Geometry check sheet. Reference: the model listing, model coordinates, mm. A direction names the side the tool comes from. Coordinates: 2 decimals unless noted, no trailing zeros. Loops run counter-clockwise (first coordinate to the right, second up) from the corner with the lowest first, then second, coordinate; pieces in that order, holes last. Notation, with made-up numbers: M 47,-35 L 64,-35 A17 ccw 64,-23 Z; hole C -7.5,57.5 d7. An arc over 180 degrees is marked long. One line per question, with ' | ' between items. Start each with the question number.
from build123d import *

# Parameters (mm, degrees)
BOSS_EXTRUDE1_DEPTH = 40
SKETCH2_R           = 15.049999999999999
CUT_EXTRUDE1_DEPTH  = 40
FILLET3_R           = 18.700000000000003
FILLET4_R           = 18.7
FILLET5_R           = 18.7
FILLET6_R           = 18.7
SKETCH4_R           = 15.049999999999999
CUT_EXTRUDE2_DEPTH  = 30


with BuildPart() as part:
    # Sketch1 → Boss-Extrude1 (new body)
    with BuildSketch(Plane.XY):
        with BuildLine():
            Line((-21.97749224689504, -20.420328952729147), (-56.618508398272695, -40.420328952728944))
            Line((-56.618508398272695, -40.420328952728944), (-74.08417498363409, -10.168907038824594))
            Line((-74.08417498363409, -10.168907038824594), (-22.896447841875652, 19.38434100567434))
            ThreePointArc((-22.896447841875652, 19.38434100567434), (1.84e-15, 30), (22.89644784187566, 19.384341005674337))
            Line((22.89644784187566, 19.384341005674337), (74.08417498363407, -10.168907038825086))
            Line((74.08417498363407, -10.168907038825086), (56.61850839827255, -40.42032895272918))
            Line((56.61850839827255, -40.42032895272918), (21.97749224689504, -20.42032895272915))
            ThreePointArc((21.97749224689504, -20.42032895272915), (-4.82e-15, -29.999999999999996), (-21.97749224689504, -20.420328952729147))
        make_face()
    extrude(amount=BOSS_EXTRUDE1_DEPTH)

    # Sketch2 → Cut-Extrude1 (cut)
    with BuildSketch(Plane(origin=(59.96639714989796, -34.62161553682567, 0), x_dir=(0, 0, -1), z_dir=(0.8660254037844382, -0.5000000000000009, 0))):
        with Locations(Location((-20, 10.769889082110701, 0), (0, 0, 90))):
            Circle(SKETCH2_R)
    cut_extrude1 = extrude(amount=-CUT_EXTRUDE1_DEPTH, mode=Mode.SUBTRACT)

    # Mirror1: Cut-Extrude1 across plane
    add(cut_extrude1.mirror(Plane(origin=(0, 0, 0), x_dir=(0, 0, 1), z_dir=(1, 0, 0))), mode=Mode.SUBTRACT)

    # Fillet3
    fillet3_edges = [part.edges().sort_by_distance(p)[0] for p in [
        (39.298000322583796, -30.420328952729164, 40),
    ]]
    fillet(fillet3_edges, radius=FILLET3_R)

    # Fillet4
    # the kernel refuses this fillet: 18.7 mm, written as the material it takes off along each edge
    with BuildSketch(Plane(origin=(-17.590239785046823, 42.759341005674386, 40), x_dir=(0, 0, -1), z_dir=(0.866025403784438, -0.5000000000000011, 0))) as fillet4_piece_1_section:
        with BuildLine():
            CenterArc((FILLET4_R, -FILLET4_R), FILLET4_R, 90, 89.99999999999997)
            Line((0, -FILLET4_R), (0, 0))
            Line((0, 0), (FILLET4_R, 0))
        make_face()
    fillet4_piece_1 = extrude(amount=152.6064960889987, mode=Mode.PRIVATE)
    fillet4_piece_1 = fillet4_piece_1 - Plane(origin=(2.66e-15, 5.33e-15, 35.12262503865641), x_dir=(-0.7632149280625219, 0.6461447001891446, 0), z_dir=(0, 0, -1)) * Cylinder(29.999999999999996, 381, mode=Mode.PRIVATE)
    add(fillet4_piece_1, mode=Mode.SUBTRACT)
    with BuildSketch(Plane(origin=(18.509195380027606, 2.9546710472706206, 0), x_dir=(-0.49999999999999495, 0.8660254037844416, 0), z_dir=(-0.8660254037844416, -0.499999999999995, 0))) as fillet4_piece_2_section:
        with BuildLine():
            CenterArc((FILLET4_R, -FILLET4_R), FILLET4_R, 90, 90)
            Line((-2.49e-15, -FILLET4_R), (0, 0))
            Line((0, 0), (FILLET4_R, 0))
        make_face()
    fillet4_piece_2 = extrude(amount=133.50000000000003, mode=Mode.PRIVATE)
    fillet4_piece_2 = fillet4_piece_2 - Plane(origin=(8.9e-16, 5.33e-15, 4.238028125601217), x_dir=(0.7325830748965012, -0.6806776317576385, 0), z_dir=(0, 0, -1)) * Cylinder(30, 342, mode=Mode.PRIVATE)
    add(fillet4_piece_2, mode=Mode.SUBTRACT)
    with BuildSketch(Plane(origin=(97.10519602519503, -63.795328952729214, 0), x_dir=(0.5000000000000009, 0.8660254037844382, 0), z_dir=(-0.8660254037844382, 0.5000000000000009, 0))) as fillet4_piece_3_section:
        with BuildLine():
            CenterArc((FILLET4_R, -FILLET4_R), FILLET4_R, 90, 90)
            Line((0, -FILLET4_R), (0, 0))
            Line((0, 0), (FILLET4_R, 0))
        make_face()
    fillet4_piece_3 = extrude(amount=133.49999999999997, mode=Mode.PRIVATE)
    fillet4_piece_3 = fillet4_piece_3 - Plane(origin=(8.9e-16, 5.33e-15, 4.238027498797153), x_dir=(0.7325830748965012, -0.6806776317576385, 0), z_dir=(0, 0, -1)) * Cylinder(30, 342, mode=Mode.PRIVATE)
    add(fillet4_piece_3, mode=Mode.SUBTRACT)

    # Fillet5
    # the kernel refuses this fillet: 18.7 mm, written as the material it takes off along each edge
    with BuildSketch(Plane(origin=(-114.57086261055673, -33.54390703882436, 0), x_dir=(0.4999999999999949, -0.8660254037844416, 0), z_dir=(0.8660254037844416, 0.49999999999999484, 0))) as fillet5_piece_1_section:
        with BuildLine():
            CenterArc((FILLET5_R, -FILLET5_R), FILLET5_R, 90, 90)
            Line((0, -FILLET5_R), (0, 0))
            Line((0, 0), (FILLET5_R, 0))
        make_face()
    fillet5_piece_1 = extrude(amount=152.6064960889985, mode=Mode.PRIVATE)
    fillet5_piece_1 = fillet5_piece_1 - Plane(origin=(8.9e-16, 5.33e-15, 4.361975698368192), x_dir=(0.7325830748965012, -0.6806776317576385, 0), z_dir=(0, 0, -1)) * Cylinder(30, 381, mode=Mode.PRIVATE)
    with BuildSketch(Plane(origin=(18.509195380027606, 2.954671047270619, 40), x_dir=(1e-17, -2e-17, -1), z_dir=(-0.8660254037844416, -0.499999999999995, 0))) as fillet5_piece_2_section:
        with BuildLine():
            CenterArc((FILLET5_R, -FILLET5_R), FILLET5_R, 90, 90)
            Line((-4.8e-16, -FILLET5_R), (0, 0))
            Line((0, 0), (FILLET5_R, 0))
        make_face()
    fillet5_piece_2 = extrude(amount=133.50000000000003, mode=Mode.PRIVATE)
    fillet5_piece_2 = fillet5_piece_2 - Plane(origin=(8.9e-16, 5.33e-15, 35.76197179193409), x_dir=(0.7325830748965012, -0.6806776317576385, 0), z_dir=(0, 0, -1)) * Cylinder(30, 342, mode=Mode.PRIVATE)
    with BuildSketch(Plane(origin=(-17.590239785046823, 42.759341005674386, 0), x_dir=(0, 0, 1), z_dir=(0.866025403784438, -0.5000000000000011, 0))) as fillet5_piece_3_section:
        with BuildLine():
            CenterArc((FILLET5_R, FILLET5_R), FILLET5_R, 180.00000000000003, 90)
            Line((-3.55e-15, FILLET5_R), (0, 0))
            Line((0, 0), (FILLET5_R, 0))
        make_face()
    fillet5_piece_3 = extrude(amount=152.6064960889987, mode=Mode.PRIVATE)
    fillet5_piece_3 = fillet5_piece_3 - Plane(origin=(8.9e-16, 5.33e-15, 4.877369917658315), x_dir=(0.7325830748965012, -0.6806776317576385, 0), z_dir=(0, 0, -1)) * Cylinder(30, 381, mode=Mode.PRIVATE)
    add([fillet5_piece_1, fillet5_piece_2, fillet5_piece_3], mode=Mode.SUBTRACT)

    # Fillet6
    # the kernel refuses this fillet: 18.7 mm, written as the material it takes off along each edge
    with BuildSketch(Plane(origin=(-114.57086261055673, -33.54390703882436, 40), x_dir=(0.4999999999999949, -0.8660254037844416, 0), z_dir=(0.8660254037844416, 0.49999999999999484, 0))) as fillet6_piece_1_section:
        with BuildLine():
            CenterArc((FILLET6_R, FILLET6_R), FILLET6_R, 180, 90)
            Line((0, FILLET6_R), (0, 0))
            Line((0, 0), (FILLET6_R, 0))
        make_face()
    fillet6_piece_1 = extrude(amount=152.6064960889985, mode=Mode.PRIVATE)
    fillet6_piece_1 = fillet6_piece_1 - Plane(origin=(8.9e-16, 5.33e-15, 35.63802430163197), x_dir=(0.7325830748965012, -0.6806776317576385, 0), z_dir=(0, 0, -1)) * Cylinder(30, 381, mode=Mode.PRIVATE)
    add(fillet6_piece_1, mode=Mode.SUBTRACT)

    # Sketch4 → Cut-Extrude2 (cut)
    with BuildSketch(Plane(origin=(0, 0, 0), x_dir=(-1, 0, 0), z_dir=(0, 0, -1))):
        Circle(SKETCH4_R)
    extrude(amount=-CUT_EXTRUDE2_DEPTH, mode=Mode.SUBTRACT)


solid = part.part
1. Draft check along X on faces 1 (the cylindrical face through (-52.079, -3.138, 33.935)), 2 (the flat face through (0, 0, 30)), 3 (the flat face through (48.132, 4.815, 19.982)). Enter one of: +X half, -X half, draft (parallel to the pull), parting line (faces both ways), or undercut.
2. Thickness scan on line 1 (X direction, y = -16, z = 4.5); line 2 (X direction, y = 2, z = 20.5); line 3 (Y direction, x = 0, z = 12). Record the ranges inside material, lowest first.
3. Depth check by flat-ended pin: pin 1 Ø6 at (x, z) = (-28.5, 30) entering from -Y; pin 2 Ø12 at (x, z) = (1, 24.5) entering from -Y; pin 3 Ø15 at (x, y) = (-3.5, 0.5) entering from -Z; pin 4 Ø10 at (x, y) = (-27, 15.5) entering from -Z. Enter the tip coordinate at first touch or a pass-through.
4. Sectioned sample at D-D (y = 0). State how many separate pieces and enclosed holes the cut face has, and give its area (3 significant figures).
5. Sectioned sample at C-C (z = 33). Record the cut outline in (x, y).
6. Sectioned sample at A-A (z = 13.5). Record the cut outline in (x, y), and give its area (3 significant figures).
7. Tool access check on faces 4 (the cylindrical face through (-40.967, -25.71, 33.935)), 5 (the cylindrical face through (3.263, -14.692, 14.79)), 6 (the cylindrical face through (41.6, -25.77, 5.78)), 7 (the flat face through (39.54, -30.56, 19.98)). Record the directions out of +Z, -Z, +X, -X, +Y, -Y that give a thin tool (end or side, any length) a straight path to the whole face; none if there is none.
8. Sectioned sample at B-B (x = 0). Record the cut outline in (y, z), and give its area (3 significant figures).
Result:
1) face 1: -X half | face 2: undercut | face 3: +X half
2) line 1: x = -70.72 to -27.39, -25.38 to 25.38, 27.39 to 70.72 | line 2: x = -53.01 to -48.16, -34.92 to -14.92, 14.92 to 34.92, 48.16 to 53.01 | line 3: y = -30 to -15.05, 15.05 to 30
3) pin 1: stops at y = -24.05 | pin 2: stops at y = -30 | pin 3: stops at z = 30 | pin 4: stops at z = 0
4) separate pieces: 1 | enclosed holes: 2 | area: 2,320 mm2
5) outline: M -72.03,-13.73 L -69.14,-18.73 L -34.5,1.27 L -26.92,-11.86 L -61.56,-31.86 L -58.67,-36.86 L -24.59,-17.18 A30 ccw 24.59,-17.18 L 58.67,-36.86 L 61.56,-31.86 L 26.92,-11.86 L 34.5,1.27 L 69.14,-18.73 L 72.03,-13.73 L 27.51,11.97 A30 ccw -27.51,11.97 Z
6) outline: M -73.72,-10.81 L -72.14,-13.54 L -37.5,6.46 L -23.92,-17.05 L -58.56,-37.05 L -56.99,-39.78 L -22.48,-19.86 A30 ccw 22.48,-19.86 L 56.99,-39.78 L 58.56,-37.05 L 23.92,-17.05 L 37.5,6.46 L 72.14,-13.54 L 73.72,-10.81 L 24.14,17.82 A30 ccw -24.14,17.82 Z; hole C 0,0 d30.1 | area: 2,850 mm2
7) face 4: +Z, -Y | face 5: -Z | face 6: -Z, -Y | face 7: +Z, -Z, -Y
8) outline: M -30,0 L -15.05,0 L -15.05,30 L 15.05,30 L 15.05,0 L 30,0 L 30,40 L -30,40 Z | area: 1,500 mm2
